Read the model definition and answer for the solid it produces. Units are mm, in the model's axes. Give positions to 0.01 mm unless a question says otherwise; leave off trailing zeros. Order: outer loops, then holes, each group sorted by start corner. A loop starts at its lowest first (then second) coordinate and runs counter-clockwise, first axis right, second up. Notation, with made-up numbers: M 65.5,-29 L 77.5,-29 A27 cw 77.5,5 Z; hole C 25,-33.75 d10. An arc over 180 degrees is marked long. One line per item, written item: value. Start each with the question number.
Autodesk Inventor part; units mm, degrees
ref_plane "YZ Plane" through (0, 0, 0) normal (1, 0, 0) x (0, 1, 0)
ref_plane "XZ Plane" through (0, 0, 0) normal (0, 1, 0) x (-1, 0, 0)
ref_plane "XY Plane" through (0, 0, 0) normal (0, 0, 1) x (1, 0, 0)
sketch "スケッチ1" plane through (0, 0, 0) normal (0, 1, 0) x (-1, 0, 0)
  line L0 (620, -125) -> (-620, -125)
  line L1 (-620, -125) -> (-620, 125)
  line L2 (-620, 125) -> (620, 125)
  line L3 (620, 125) -> (620, -125)
  line L4 (0, -175) -> (0, 175)
  line L5 (868, 0) -> (-868, 0)
  point P0 (0, 0)
  point P1 (0, -125)
  point P2 (620, 0)
  dimension "d0" = 1240
  dimension "d1" = 250
extrude "押し出し1" add sketch "スケッチ1" along normal blind 10
sketch "スケッチ2" plane through (0, 10, 0) normal (0, 1, 0) x (1, 0, 0)
  line L0 (0, 175) -> (0, -175)
  line L1 (0, 45) -> (200, 45)
  line L2 (200, 45) -> (520, 125)
  line L3 (620, 125) -> (-620, 125)
  line L4 (0, 45) -> (-200, 45)
  line L5 (-200, 45) -> (-520, 125)
  line L6 (620, -125) -> (620, 125)
  line L7 (-520, 125) -> (520, 125)
  line L8 (-620, -125) -> (620, -125)
  point P0 (0, 0)
  dimension "d5" = 200
  dimension "d6" = 100
  dimension "d10" = 170
extrude "押し出し2" cut sketch "スケッチ2" against normal through all contours L3 L2 L1 L0 | L0 L4 L5 L3
fillet "フィレット1" radius 500 4 edges at (-520, 5, -125) (-200, 5, -45) (200, 5, -45) (520, 5, -125)
properties part number "type7_base" material "CFRP"
Q1. This flat-tipped pin is pushed along its axis until it touches: pin 1 (3 mm diameter, centred on x = -55, y = 4, fed in from -Z). Where does it stop, or does it pass through?
Q2. Find section C-C, the plane x = 12. Give the vertices of the cut face in (y, z), then the cut area to 3 significant figures.
Q3. Find section A-A, the plane y = 1.5. Give the vertices of the cut face in (x, z) (3 decimals), then the cut area to 3 significant figures.
Q4. Determine the mould class of faces 1 (the flat face through (9, 0, 30)), 2 (the flat face through (358.6, 5.07, -84.65)), 3 (the flat face through (-358.6, 5.07, -84.65)) for opening direction X: released by +X, released by -X, zero draft, split by the parting line, or undercut.
Q5. Find section B-B, the plane x = -398. Give the vertices of the cut face in (y, z), then the cut area to 4 significant figures.
Q6. Consider probe 1 along Z at (x, y) = (150.5, 7.75); probe 2 along Z at (x, y) = (81, 3.75). Determine where each line is inside the solid, lowest interval first.
Evaluation:
1. pin 1: z = -45
2. outline: M 0,-45 L 10,-45 L 10,125 L 0,125 Z
2. area: 1,700 mm2
3. outline: M -620,-125 L -581.553,-125 A500 ccw -460.285,-110.071 L -259.715,-59.929 A500 cw -138.447,-45 L 138.447,-45 A500 cw 259.715,-59.929 L 460.285,-110.071 A500 ccw 581.553,-125 L 620,-125 L 620,125 L -620,125 Z
3. area: 252,000 mm2
4. face 1: zero draft
4. face 2: undercut
4. face 3: undercut
5. outline: M 0,-94.5 L 10,-94.5 L 10,125 L 0,125 Z
5. area: 2,195 mm2
6. probe 1: -45.15 to 125
6. probe 2: -45 to 125
